from build123d import *

# Parameters (mm, degrees)
SKETCH1_R              = 6.35
TOFITINTOBEARING_DEPTH = 12.7
SKETCH2_R              = 19.05
TOSITATOPBEARING_DEPTH = 12.7
BOSS_EXTRUDE3_START    = 6.35
BOSS_EXTRUDE3_DEPTH    = 6.35
SKETCH8_R              = 12.7
CUT_EXTRUDE3_DEPTH     = 6.35


with BuildPart() as part:
    # Sketch1 → ToFitIntoBearing (new body)
    with BuildSketch(Plane(origin=(0, 0, 0), x_dir=(1, 0, 0), z_dir=(0, 1, 0))):
        with Locations(Location((0, 0, 0), (0, 0, 270))):
            Circle(SKETCH1_R)
    extrude(amount=TOFITINTOBEARING_DEPTH)

    # Sketch2 → ToSitAtopBearing (add)
    with BuildSketch(Plane(origin=(0, 12.7, 0), x_dir=(1, 0, 0), z_dir=(0, 1, 0))):
        with Locations(Location((0, 0, 0), (0, 0, 270))):
            Circle(SKETCH2_R)
    extrude(amount=TOSITATOPBEARING_DEPTH)

    # Sketch7 → Boss-Extrude3 (add)
    with BuildSketch(Plane(origin=(0, 0, 0), x_dir=(0, 0, -1), z_dir=(1, 0, 0)).offset(BOSS_EXTRUDE3_START)):
        with BuildLine():
            Line((-19.05, 44.45), (-19.05, 25.4))
            Line((-19.05, 25.4), (19.05, 25.4))
            Line((19.05, 25.4), (19.05, 44.45))
            ThreePointArc((19.05, 44.45), (0, 63.5), (-19.05, 44.45))
        make_face()
    boss_extrude3 = extrude(amount=BOSS_EXTRUDE3_DEPTH)

    # Sketch8 → Cut-Extrude3 (cut)
    with BuildSketch(Plane.ZY.offset(-6.35)):
        with Locations((0, 44.45)):
            Circle(SKETCH8_R)
    cut_extrude3 = extrude(amount=-CUT_EXTRUDE3_DEPTH, mode=Mode.SUBTRACT)

    # Mirror2: Boss-Extrude3, Cut-Extrude3 across plane
    add(boss_extrude3.mirror(Plane(origin=(0, 0, 0), x_dir=(0, 0, 1), z_dir=(1, 0, 0))))
    add(cut_extrude3.mirror(Plane(origin=(0, 0, 0), x_dir=(0, 0, 1), z_dir=(1, 0, 0))), mode=Mode.SUBTRACT)


solid = part.part
Work out the finished part from the listing and answer in its coordinate system (mm). A direction names the side the tool comes from. Give positions to 0.01 mm unless a question says otherwise; leave off trailing zeros. Loops run counter-clockwise (first coordinate to the right, second up) from the corner with the lowest first, then second, coordinate; pieces in that order, holes last. Notation, with made-up numbers: (45, 36.25) -> (92, 36.25) arc R18 cw to (92, 51.25) -> close; hole circle Ø11 at (44.25, 41.25). An arc over 180 degrees is marked (long way). Use a Markdown table: item, result. Add a question column.
1) The part is cut by section B-B, the plane x = 0. Determine the outline of the cut face in (y, z).
2) The part is cut by section D-D, the plane x = -12. Determine the outline of the cut face in (y, z), plus the area to 3 significant figures.
3) Consider line 1 along Y through (x, z) = (10.5, 0); line 2 along Z through (x, y) = (9, 44); line 3 along X through (y, z) = (33, -9). Determine where each line is inside the solid, lowest interval first.
4) The part is cut by section C-C, the plane y = 21. Determine the outline of the cut face in (x, z).
5) Which of the six approach directions +Z, -Z, +X, -X, +Y, -Y give full straight-line access (tool end or side, diameter ignored) to faces 1 (the flat face through (-10, 25.4, -18)), 2 (the flat face through (12.7, 32, -4)), 3 (the flat face through (10, 25.4, 18)), 4 (the flat face through (5, 12.7, -5)), 5 (the flat face through (-15, 25.4, 0))?
6) For a pull along X with two mould halves and no side action, classify faces 6 (the flat face through (9, 35, 19.05)), 7 (the flat face through (6.35, 32, -4)), 8 (the flat face through (-12.7, 32, -4)) as +X half, -X half, draft (parallel to the pull), parting line (faces both ways), or undercut.
7) The part is cut by section A-A, the plane z = 0. Determine the outline of the cut face in (x, y), plus the area to 3 significant figures.
8) Each of these flat-tipped pins is pushed along its axis until it touches: P1, Ø8, axis at y = 16, z = -11.5, coming from the -X side; P2, Ø12, axis at x = 12.5, z = 3, coming from the -Y side; P3, Ø3, axis at x = 17.5, z = -0.5, coming from the +Y side. Where does it stop, or does it pass through?
Reported:
| question | item | result |
|---|---|---|
| 1 | outline | (0, -6.35) -> (12.7, -6.35) -> (12.7, -19.05) -> (25.4, -19.05) -> (25.4, 19.05) -> (12.7, 19.05) -> (12.7, 6.35) -> (0, 6.35) -> close |
| 2 | outline | (12.7, -14.8) -> (25.4, -14.8) -> (25.4, -19.05) -> (44.45, -19.05) arc R19.05 ccw to (44.45, 19.05) -> (25.4, 19.05) -> (25.4, 14.8) -> (12.7, 14.8) -> close; hole circle Ø25.4 at (44.45, 0) |
| 2 | area | 1,160 mm^2 |
| 3 | line 1 | y = 12.7 to 31.75, 57.15 to 63.5 |
| 3 | line 2 | z = -19.05 to -12.69, 12.69 to 19.05 |
| 3 | line 3 | x = -12.7 to -6.35, 6.35 to 12.7 |
| 4 | outline | circle Ø38.1 at (0, 0) |
| 5 | face 1 | -Z, -X, -Y |
| 5 | face 2 | +Z, -Z, +X, +Y |
| 5 | face 3 | +Z, +X, -Y |
| 5 | face 4 | -Y |
| 5 | face 5 | +Z, -Z, -X, +Y |
| 6 | face 6 | draft |
| 6 | face 7 | undercut |
| 6 | face 8 | -X half |
| 7 | outline | (-19.05, 12.7) -> (-6.35, 12.7) -> (-6.35, 0) -> (6.35, 0) -> (6.35, 12.7) -> (19.05, 12.7) -> (19.05, 25.4) -> (12.7, 25.4) -> (12.7, 31.75) -> (6.35, 31.75) -> (6.35, 25.4) -> (-6.35, 25.4) -> (-6.35, 31.75) -> (-12.7, 31.75) -> (-12.7, 25.4) -> (-19.05, 25.4) -> close; (-12.7, 57.15) -> (-6.35, 57.15) -> (-6.35, 63.5) -> (-12.7, 63.5) -> close; (6.35, 57.15) -> (12.7, 57.15) -> (12.7, 63.5) -> (6.35, 63.5) -> close |
| 7 | area | 806 mm^2 |
| 8 | P1 | stops at x = -17.51 |
| 8 | P2 | stops at y = 12.7 |
| 8 | P3 | stops at y = 25.4 |
